Geometry: final body of the model. Coordinates: model frame, mm. Coordinates: 2 decimals unless noted, no trailing zeros. Loops run counter-clockwise (first coordinate to the right, second up) from the corner with the lowest first, then second, coordinate; pieces in that order, holes last. Notation, with made-up numbers: (49, 89.25) - (77, 89.25) arc R25 ccw to (77, 101.25) - close; hole circle Ø7 at (47.5, 38). An arc over 180 degrees is marked (long way). Return JSON: item names as keys, results as strings.
from build123d import *

# Parameters (mm, degrees)
F0_W         = 37
F0_H         = 15
F1_DEPTH     = 17
F2_R         = 5.75
F3_DEPTH     = 7
F6_T1_DEPTH  = 44.5
F6_T3_DEPTH  = 42
F6_T5_DEPTH  = 7
F6_T7_DEPTH  = 5
F6_S11_W     = 5
F6_S11_H     = 5
F6_T12_DEPTH = 5
F6_S17_W     = 5
F6_S17_H     = 5
F6_T18_DEPTH = 5
F6_S23_W     = 5
F6_S23_H     = 5
F6_T24_DEPTH = 5
F6_S29_W     = 5
F6_S29_H     = 5
F6_T30_DEPTH = 5


# Not quite as in the source:
# - a fillet or chamfer that OpenCascade refuses, or shapes differently, is made with other operations: its cross-section is extruded or revolved along the edge and cut away or added


with BuildPart() as f1:
    # F0 (on Front) → F1 (new body)
    with BuildSketch(Plane.XZ):
        Rectangle(F0_W, F0_H)
    extrude(amount=F1_DEPTH)

    # F2 (on face) → F3 (cut)
    with BuildSketch(Plane.XZ.offset(17)):
        with Locations((8.75, 0)):
            Circle(F2_R)
    extrude(amount=-F3_DEPTH, mode=Mode.SUBTRACT)

    # F4 (on face) → F5 (revolve, cut)
    with BuildSketch(Plane.XZ.offset(10)):
        with BuildLine():
            Line((8.75, 0), (8.75, 5.75))
            ThreePointArc((8.75, 5.75), (3, 0), (8.75, -5.75))
            Line((8.75, -5.75), (8.75, 0))
        make_face()
    revolve(axis=Axis((8.75, -10, 2.875), (0, 0, 1)), mode=Mode.SUBTRACT)

    # F6: fillet of radius 5 on 10 edges, made by hand

    # F6_s2 → F6_t1 (cut)
    with BuildSketch(Plane.YZ.offset(-13.5)):
        with BuildLine():
            ThreePointArc((-17, 2.5), (-15.5355339059, 6.0355339059), (-12, 7.5))
            Line((-12, 7.5), (-17, 7.5))
            Line((-17, 7.5), (-17, 2.5))
        make_face()
        with BuildLine():
            ThreePointArc((-12, -7.5), (-15.5355339059, -6.0355339059), (-17, -2.5))
            Line((-17, -2.5), (-17, -7.5))
            Line((-17, -7.5), (-12, -7.5))
        make_face()
        with BuildLine():
            ThreePointArc((0, 2.5), (-1.4644660941, 6.0355339059), (-5, 7.5))
            Line((-5, 7.5), (0, 7.5))
            Line((0, 7.5), (0, 2.5))
        make_face()
        with BuildLine():
            ThreePointArc((-5, -7.5), (-1.4644660941, -6.0355339059), (0, -2.5))
            Line((0, -2.5), (0, -7.5))
            Line((0, -7.5), (-5, -7.5))
        make_face()
    extrude(amount=F6_T1_DEPTH, mode=Mode.SUBTRACT)

    # F6_s4 → F6_t3 (cut)
    with BuildSketch(Plane.XZ.offset(-12.5)):
        with BuildLine():
            ThreePointArc((18.5, 2.5), (17.0355339059, 6.0355339059), (13.5, 7.5))
            Line((13.5, 7.5), (18.5, 7.5))
            Line((18.5, 7.5), (18.5, 2.5))
        make_face()
        with BuildLine():
            ThreePointArc((13.5, -7.5), (17.0355339059, -6.0355339059), (18.5, -2.5))
            Line((18.5, -2.5), (18.5, -7.5))
            Line((18.5, -7.5), (13.5, -7.5))
        make_face()
    extrude(amount=F6_T3_DEPTH, mode=Mode.SUBTRACT)

    # F6_s6 → F6_t5 (cut)
    with BuildSketch(Plane.XZ.offset(5)):
        with BuildLine():
            ThreePointArc((-18.5, 2.5), (-17.0355339059, 6.0355339059), (-13.5, 7.5))
            Line((-13.5, 7.5), (-18.5, 7.5))
            Line((-18.5, 7.5), (-18.5, 2.5))
        make_face()
        with BuildLine():
            ThreePointArc((-13.5, -7.5), (-17.0355339059, -6.0355339059), (-18.5, -2.5))
            Line((-18.5, -2.5), (-18.5, -7.5))
            Line((-18.5, -7.5), (-13.5, -7.5))
        make_face()
    extrude(amount=F6_T5_DEPTH, mode=Mode.SUBTRACT)

    # F6_s8 → F6_t7 (cut)
    with BuildSketch(Plane.XY.offset(-2.5)):
        with BuildLine():
            ThreePointArc((-18.5, -12), (-17.0355339059, -15.5355339059), (-13.5, -17))
            Line((-13.5, -17), (-18.5, -17))
            Line((-18.5, -17), (-18.5, -12))
        make_face()
        with BuildLine():
            ThreePointArc((-18.5, -5), (-17.0355339059, -1.4644660941), (-13.5, 0))
            Line((-13.5, 0), (-18.5, 0))
            Line((-18.5, 0), (-18.5, -5))
        make_face()
    extrude(amount=F6_T7_DEPTH, mode=Mode.SUBTRACT)


with BuildPart() as f6_tool10:
    # F6_s11 → F6_t12 (new body)
    with BuildSketch(Plane.YZ.offset(-13.5)):
        with Locations((-14.5, 5)):
            Rectangle(F6_S11_W, F6_S11_H)
    extrude(amount=-F6_T12_DEPTH)

    # F6_s13 → F6_t14 (revolve, cut)
    with BuildSketch(Plane(origin=(-13.5, -12, 2.5), x_dir=(0, 0.7071067812, -0.7071067812), z_dir=(0, 0.7071067812, 0.7071067812))):
        with BuildLine():
            ThreePointArc((0, -5), (5, 0), (0, 5))
            Line((0, 5), (0, -5))
        make_face()
    revolve(axis=Axis((-13.5, -12, 2.5), (-1, 0, 0)), mode=Mode.SUBTRACT)


with BuildPart() as f1_1:
    add(f1.part)

    # F6_t9: cut F6_tool10
    add(f6_tool10.part, mode=Mode.SUBTRACT)


with BuildPart() as f6_tool16:
    # F6_s17 → F6_t18 (new body)
    with BuildSketch(Plane.XY.offset(-2.5)):
        with Locations((-16, -14.5)):
            Rectangle(F6_S17_W, F6_S17_H)
    extrude(amount=-F6_T18_DEPTH)

    # F6_s19 → F6_t20 (revolve, cut)
    with BuildSketch(Plane(origin=(-13.5, -12, -2.5), x_dir=(0.7071067812, 0.7071067812, 0), z_dir=(-0.7071067812, 0.7071067812, 0))):
        with BuildLine():
            ThreePointArc((0, -5), (5, 0), (0, 5))
            Line((0, 5), (0, -5))
        make_face()
    revolve(axis=Axis((-13.5, -12, -2.5), (0, 0, -1)), mode=Mode.SUBTRACT)


with BuildPart() as f1_2:
    add(f1_1.part)

    # F6_t15: cut F6_tool16
    add(f6_tool16.part, mode=Mode.SUBTRACT)


with BuildPart() as f6_tool22:
    # F6_s23 → F6_t24 (new body)
    with BuildSketch(Plane.YZ.offset(-13.5)):
        with Locations((-2.5, 5)):
            Rectangle(F6_S23_W, F6_S23_H)
    extrude(amount=-F6_T24_DEPTH)

    # F6_s25 → F6_t26 (revolve, cut)
    with BuildSketch(Plane(origin=(-13.5, -5, 2.5), x_dir=(0, -0.7071067812, -0.7071067812), z_dir=(0, 0.7071067812, -0.7071067812))):
        with BuildLine():
            ThreePointArc((0, -5), (5, 0), (0, 5))
            Line((0, 5), (0, -5))
        make_face()
    revolve(axis=Axis((-13.5, -5, 2.5), (-1, 0, 0)), mode=Mode.SUBTRACT)


with BuildPart() as f1_3:
    add(f1_2.part)

    # F6_t21: cut F6_tool22
    add(f6_tool22.part, mode=Mode.SUBTRACT)


with BuildPart() as f6_tool28:
    # F6_s29 → F6_t30 (new body)
    with BuildSketch(Plane.XY.offset(-2.5)):
        with Locations((-16, -2.5)):
            Rectangle(F6_S29_W, F6_S29_H)
    extrude(amount=-F6_T30_DEPTH)

    # F6_s31 → F6_t32 (revolve, cut)
    with BuildSketch(Plane(origin=(-13.5, -5, -2.5), x_dir=(0.7071067812, -0.7071067812, 0), z_dir=(0.7071067812, 0.7071067812, 0))):
        with BuildLine():
            ThreePointArc((0, -5), (5, 0), (0, 5))
            Line((0, 5), (0, -5))
        make_face()
    revolve(axis=Axis((-13.5, -5, -2.5), (0, 0, -1)), mode=Mode.SUBTRACT)


with BuildPart() as f1_4:
    add(f1_3.part)

    # F6_t27: cut F6_tool28
    add(f6_tool28.part, mode=Mode.SUBTRACT)


solid = f1_4.part
Item 1: Ray query, probe 1 along Z at (x, y) = (8.75, -12); probe 2 along X at (y, z) = (-12, 0); probe 3 along X at (y, z) = (-15.5, -4.25). Return the intervals inside material, ascending. Write a range as from..to.
Worked out:
{"probe 1": "-7.5..-5.75, 5.75..7.5", "probe 2": "-18.5..3, 14.5..18.5", "probe 3": "-16.61..4.88, 12.62..18.18"}
Item 2: First-contact query: pin 1 Ø6 at (y, z) = (-15, 4) entering from -X. Flat tip, straight axial feed; report the tip coordinate or a pass-through.
Worked out:
{"pin 1": "x = -18.49"}
Item 3: Mould query, pull axis Z, two halves, no side actions, for faces 1 (the face through (7.504, -13.549, -5.613)), 2 (the face through (2.28, -1.5, -6.07)), 3 (the face through (2.28, -1.43, 6)), 4 (the face through (2, 0, 0)). Classes: +Z half, -Z half, draft (parallel to the pull), parting line (faces both ways), or undercut.
Worked out:
{"face 1": "undercut", "face 2": "-Z half", "face 3": "+Z half", "face 4": "draft"}
Item 4: Section query B-B, the plane y = -11. Return loops of the section in (x, z).
Worked out:
{"outline": "(-18.5, -2.5) arc R5 ccw to (-13.5, -7.5) - (13.5, -7.5) arc R5 ccw to (18.5, -2.5) - (18.5, 2.5) arc R5 ccw to (13.5, 7.5) - (-13.5, 7.5) arc R5 ccw to (-18.5, 2.5) - close; hole circle Ø11.5 at (8.75, 0)"}
Item 5: Section query D-D, the plane y = -9. Return loops of the section in (x, z), and give its area (3 significant figures).
Worked out:
{"outline": "(-18.5, -2.5) arc R5 ccw to (-13.5, -7.5) - (13.5, -7.5) arc R5 ccw to (18.5, -2.5) - (18.5, 2.5) arc R5 ccw to (13.5, 7.5) - (-13.5, 7.5) arc R5 ccw to (-18.5, 2.5) - close; hole circle Ø11.32 at (8.75, 0)", "area": "433 mm^2"}
Item 6: Section query A-A, the plane z = 0. Return loops of the section in (x, y).
Worked out:
{"outline": "(-18.5, -12) arc R5 ccw to (-13.5, -17) - (3, -17) - (3, -10) arc R5.75 cw to (14.5, -10) - (14.5, -17) - (18.5, -17) - (18.5, 0) - (-13.5, 0) arc R5 ccw to (-18.5, -5) - close"}
Item 7: Section query C-C, the plane x = 16.5. Return loops of the section in (y, z), and give its area (3 significant figures).
Worked out:
{"outline": "(-17, -2.5) arc R5 ccw to (-15, -6.5) - (-2, -6.5) arc R5 ccw to (0, -2.5) - (0, 2.5) arc R5 ccw to (-2, 6.5) - (-15, 6.5) arc R5 ccw to (-17, 2.5) - close", "area": "211 mm^2"}
